Geometry check sheet. Reference: the model listing, model coordinates, mm. A direction names the side the tool comes from. Coordinates: 2 decimals unless noted, no trailing zeros. Write each loop counter-clockwise with the first axis right and the second up, starting at its lowest first coordinate (ties: lowest second). Pieces come first, ordered by that corner, then holes. Notation, with made-up numbers: (30.25, 24) -> (86.25, 24) arc R26 cw to (86.25, 43) -> close; hole circle Ø2 at (2, 63). An arc over 180 degrees is marked (long way). Answer in a Markdown table with one row per item. Add a question column.
Q1. Gauge pin test, flat ends, axial feed: P1, Ø1.8, axis at x = 15, y = 0, coming from the -Z side; P2, Ø3, axis at y = -2, z = 4, coming from the +X side. Record the tip position at first contact, or that the pin passes through.
Q2. Release check for a two-part mould opening along X. For faces 1 (the face through (-8, 0, 5)), 2 (the face through (-16.5, 0.07, 2.46)), 3 (the face through (18.635, -0.063, 4.865)) record: pulls with the +X half, pulls with the -X half, needs draft (parallel to the pull), parting line crosses it, or undercut.
Q3. Section check B-B, the plane y = 0. Record the boundary of the cut face in (x, z), and give its area (3 significant figures).
Q4. Tool access check on faces 4 (the face through (-9.489, 5.922, 4.754)), 5 (the face through (-7.493, 0.33, 5.493)). Record the directions out of +Z, -Z, +X, -X, +Y, -Y that give a thin tool (end or side, any length) a straight path to the whole face; none if there is none.
Q5. Section check C-C, the plane z = 2.7. Record the boundary of the cut face in (x, y), and give its area (3 significant figures).
Q6. Section check D-D, the plane z = 5.65. Record the boundary of the cut face in (x, y), and give its area (3 significant figures).
Q7. Section check A-A, the plane x = 0. Record the boundary of the cut face in (y, z).
Q8. Thickness scan on line 1 (Y direction, x = 0, z = 2.45); line 2 (Z direction, x = 3, y = 7.5); line 3 (Y direction, x = -15, z = 1.45). Record the ranges inside material, lowest first.
```python
from build123d import *

# Parameters (mm, degrees)
F0_R     = 1.5
F1_DEPTH = 5
F2_R     = 1.5
F3_DEPTH = 5.001
F4_R     = 2
F5_DEPTH = 4
F6_R     = 7.5
F6_R_2   = 1.5
F7_DEPTH = 1
F8_SIZE  = 0.5


with BuildPart() as f1:
    # F0 (on Top) → F1 (new body)
    with BuildSketch(Plane.XY):
        with BuildLine():
            Line((-3, 8.485281), (-16.333333, 3.771236))
            ThreePointArc((-16.333333, 3.771236), (-19, 0), (-16.333333, -3.771236))
            Line((-16.333333, -3.771236), (-3, -8.485281))
            ThreePointArc((-3, -8.485281), (0, -9), (3, -8.485281))
            Line((3, -8.485281), (16.333333, -3.771236))
            ThreePointArc((16.333333, -3.771236), (19, 0), (16.333333, 3.771236))
            Line((16.333333, 3.771236), (3, 8.485281))
            ThreePointArc((3, 8.485281), (0, 9), (-3, 8.485281))
        make_face()
        with Locations((-15, 0)):
            Circle(F0_R, mode=Mode.SUBTRACT)
        with Locations((15, 0)):
            Circle(F0_R, mode=Mode.SUBTRACT)
    extrude(amount=F1_DEPTH)

    # F2 (on face) → F3 (cut, through all)
    with BuildSketch(Plane(origin=(0, 0, 0), x_dir=(1, 0, 0), z_dir=(0, 0, -1))):
        Circle(F2_R)
    extrude(amount=-F3_DEPTH, mode=Mode.SUBTRACT)

    # F4 (on face) → F5 (cut)
    with BuildSketch(Plane(origin=(0, 0, 0), x_dir=(1, 0, 0), z_dir=(0, 0, -1))):
        Circle(F4_R)
    extrude(amount=-F5_DEPTH, mode=Mode.SUBTRACT)

    # F6 (on face) → F7 (join)
    with BuildSketch(Plane.XY.offset(5)):
        Circle(F6_R)
        Circle(F6_R_2, mode=Mode.SUBTRACT)
    extrude(amount=F7_DEPTH)

    # F8
    f8_edges = [f1.edges().sort_by_distance(p)[0] for p in [
        (9.666667, 6.128259, 5),
    ]]
    chamfer(f8_edges, length=F8_SIZE)


solid = f1.part
```
Calculated:
| question | item | result |
|---|---|---|
| 1 | P1 | passes through |
| 1 | P2 | stops at x = 18.97 |
| 2 | face 1 | needs draft |
| 2 | face 2 | undercut |
| 2 | face 3 | pulls with the +X half |
| 3 | outline | (-19, 0) -> (-16.5, 0) -> (-16.5, 5) -> (-18.5, 5) -> (-19, 4.5) -> close; (-13.5, 0) -> (-2, 0) -> (-2, 4) -> (-1.5, 4) -> (-1.5, 6) -> (-7.5, 6) -> (-7.5, 5) -> (-13.5, 5) -> close; (1.5, 4) -> (2, 4) -> (2, 0) -> (13.5, 0) -> (13.5, 5) -> (7.5, 5) -> (7.5, 6) -> (1.5, 6) -> close; (16.5, 0) -> (19, 0) -> (19, 4.5) -> (18.5, 5) -> (16.5, 5) -> close |
| 3 | area | 153 mm² |
| 4 | face 4 | +Z, -X, +Y |
| 4 | face 5 | +Z |
| 5 | outline | (-16.33, -3.77) -> (-3, -8.49) arc R9 ccw to (3, -8.49) -> (16.33, -3.77) arc R4 ccw to (16.33, 3.77) -> (3, 8.49) arc R9 ccw to (-3, 8.49) -> (-16.33, 3.77) arc R4 ccw to start; hole circle Ø3 at (-15, 0); hole circle Ø4 at (0, 0); hole circle Ø3 at (15, 0) |
| 5 | area | 435 mm² |
| 6 | outline | circle Ø15 at (0, 0); hole circle Ø3 at (0, 0) |
| 6 | area | 170 mm² |
| 7 | outline | (-9, 0) -> (-2, 0) -> (-2, 4) -> (-1.5, 4) -> (-1.5, 6) -> (-7.5, 6) -> (-7.5, 5) -> (-8.5, 5) -> (-9, 4.5) -> close; (1.5, 4) -> (2, 4) -> (2, 0) -> (9, 0) -> (9, 4.5) -> (8.5, 5) -> (7.5, 5) -> (7.5, 6) -> (1.5, 6) -> close |
| 8 | line 1 | y = -9 to -2, 2 to 9 |
| 8 | line 2 | z = 0 to 5 |
| 8 | line 3 | y = -4.24 to -1.5, 1.5 to 4.24 |
